Design review of the part built by this model. Coordinates are the model's own, in mm. A direction names the side the tool comes from. Round coordinates to 2 decimals unless told otherwise and drop trailing zeros. Loops run counter-clockwise (first coordinate to the right, second up) from the corner with the lowest first, then second, coordinate; pieces in that order, holes last. Notation, with made-up numbers: (26.5, 36) - (46.5, 36) arc R10 cw to (46.5, 41) - close; hole circle Ø3 at (8.25, 42). An arc over 180 degrees is marked (long way). Return JSON: item names as keys, results as strings. Group by question number.
(1) For faces 1 (the flat face through (15, 0, -1)), 2 (the cylindrical face through (13.02, 1.48, -12.79)), list the 3-axis set-ups (+Z, -Z, +X, -X, +Y, -Y) from which the entire face can be reached by the end or side of a thin tool; tool diameter is ignored.
(2) We need section B-B, the plane y = 2.3. Write out the cut boundary in (x, z), and give its area (3 significant figures).
(3) We need section C-C, the plane z = 21. Write out the cut boundary in (x, y), and give its area (3 significant figures).
(4) We need section D-D, the plane x = 37.5. Write out the cut boundary in (y, z), and give its area (3 significant figures).
(5) The part is to be moulded in two halves that separate along X. For faces 3 (the flat face through (2.5, 1, 21)), 4 (the flat face through (15, 3, -1)), 5 (the flat face through (6.5, 2, -42)), say which applies: pulls with the +X half, pulls with the -X half, needs draft (parallel to the pull), parting line crosses it, or undercut.
(6) We need section A-A, the plane x = 0. Write out the cut boundary in (y, z).
(7) Clearance check with flat-ended pins moving along their axes: pin 1 (0.9 mm diameter, centred on y = 1.5, z = -21.5, fed in from -X); pin 2 (1.5 mm diameter, centred on x = 21, y = 2, fed in from +Z); pin 3 (0.9 mm diameter, centred on y = 1.5, z = -20.5, fed in from +X). State where each tip first meets the part, or that it passes through.
(8) Wall thickness on L1, parallel to X at y = 0.35, z = -5.5; L2, parallel to X at y = 1.9, z = 0; L3, parallel to Z at x = -16, y = 2.9: over which ranges is each line inside the solid? List them lowest first. Write a range as [from, to].
from build123d import *

# Parameters (mm, degrees)
SKETCH1_R           = 62.5
SKETCH1_R_2         = 13.25
BOSS_EXTRUDE1_DEPTH = 3
CUT_EXTRUDE1_DEPTH  = 89.439244682


with BuildPart() as part:
    # Sketch1 → Boss-Extrude1 (new body)
    with BuildSketch(Plane(origin=(0, 0, 0), x_dir=(1, 0, 0), z_dir=(0, 1, 0))):
        with Locations(Location((0, 0, 0), (0, 0, 270))):
            Circle(SKETCH1_R)
        with Locations(Location((0, 0, 0), (0, 0, 270))):
            Circle(SKETCH1_R_2, mode=Mode.SUBTRACT)
        with BuildLine():
            Line((-2.5, 18.07795619), (-2.5, 23.115200626))
            ThreePointArc((-2.5, 23.115200626), (-16.440232663, 16.440232663), (-23.115200626, 2.5))
            Line((-23.115200626, 2.5), (-18.07795619, 2.5))
            ThreePointArc((-18.07795619, 2.5), (-12.904698757, 12.904698757), (-2.5, 18.07795619))
        make_face(mode=Mode.SUBTRACT)
        with BuildLine():
            Line((2.5, 18.07795619), (2.5, 23.115200626))
            ThreePointArc((2.5, 23.115200626), (16.440232663, 16.440232663), (23.115200626, 2.5))
            Line((23.115200626, 2.5), (18.07795619, 2.5))
            ThreePointArc((18.07795619, 2.5), (12.904698757, 12.904698757), (2.5, 18.07795619))
        make_face(mode=Mode.SUBTRACT)
        with BuildLine():
            Line((18.07795619, -2.5), (23.115200626, -2.5))
            ThreePointArc((23.115200626, -2.5), (16.440232663, -16.440232663), (2.5, -23.115200626))
            Line((2.5, -23.115200626), (2.5, -18.07795619))
            ThreePointArc((2.5, -18.07795619), (12.904698757, -12.904698757), (18.07795619, -2.5))
        make_face(mode=Mode.SUBTRACT)
        with BuildLine():
            Line((-2.5, -18.07795619), (-2.5, -23.115200626))
            ThreePointArc((-2.5, -23.115200626), (-16.440232663, -16.440232663), (-23.115200626, -2.5))
            Line((-23.115200626, -2.5), (-18.07795619, -2.5))
            ThreePointArc((-18.07795619, -2.5), (-12.904698757, -12.904698757), (-2.5, -18.07795619))
        make_face(mode=Mode.SUBTRACT)
    extrude(amount=BOSS_EXTRUDE1_DEPTH)

    # Sketch4 → Cut-Extrude1 (cut, through all)
    with BuildSketch(Plane(origin=(0, 3, 0), x_dir=(1, 0, 0), z_dir=(0, 1, 0))):
        with BuildLine():
            Line((-6.5, 31.7), (-6.5, 52.3))
            ThreePointArc((-6.5, 52.3), (0, 58.8), (6.5, 52.3))
            Line((6.5, 52.3), (6.5, 31.7))
            ThreePointArc((6.5, 31.7), (0, 25.2), (-6.5, 31.7))
        make_face()
    extrude(amount=-CUT_EXTRUDE1_DEPTH, mode=Mode.SUBTRACT)


solid = part.part
Solutions:
{
 "1": {"face 1": "+Z, -Z, +X, -X, -Y", "face 2": "+Y, -Y"},
 "2": {"outline": "circle Ø125 at (0, 0); hole (-23.12, -2.5) arc R23.25 ccw to (-2.5, -23.12) - (-2.5, -18.08) arc R18.25 cw to (-18.08, -2.5) - close; hole (-23.12, 2.5) - (-18.08, 2.5) arc R18.25 cw to (-2.5, 18.08) - (-2.5, 23.12) arc R23.25 ccw to start; hole circle Ø26.5 at (0, 0); hole (-6.5, -52.3) arc R6.5 ccw to (6.5, -52.3) - (6.5, -31.7) arc R6.5 ccw to (-6.5, -31.7) - close; hole (2.5, -23.12) arc R23.25 ccw to (23.12, -2.5) - (18.08, -2.5) arc R18.25 cw to (2.5, -18.08) - close; hole (2.5, 18.08) arc R18.25 cw to (18.08, 2.5) - (23.12, 2.5) arc R23.25 ccw to (2.5, 23.12) - close", "area": "10,800 mm^2"},
 "3": {"outline": "(-58.87, 0) - (-9.98, 0) - (-9.98, 3) - (-58.87, 3) - close; (-2.5, 0) - (2.5, 0) - (2.5, 3) - (-2.5, 3) - close; (9.98, 0) - (58.87, 0) - (58.87, 3) - (9.98, 3) - close", "area": "308 mm^2"},
 "4": {"outline": "(0, -50) - (3, -50) - (3, 50) - (0, 50) - close", "area": "300 mm^2"},
 "5": {"face 3": "undercut", "face 4": "needs draft", "face 5": "undercut"},
 "6": {"outline": "(0, -62.5) - (3, -62.5) - (3, -58.8) - (0, -58.8) - close; (0, -25.2) - (3, -25.2) - (3, -13.25) - (0, -13.25) - close; (0, 13.25) - (3, 13.25) - (3, 62.5) - (0, 62.5) - close"},
 "7": {"pin 1": "x = -58.85", "pin 2": "z = 59.13", "pin 3": "x = 59.2"},
 "8": {"L1": "[-62.26, -22.59], [-17.4, -12.05], [12.05, 17.4], [22.59, 62.26]", "L2": "[-62.5, -13.25], [13.25, 62.5]", "L3": "[-60.42, -16.87], [-8.78, 8.78], [16.87, 60.42]"}
}
